```python
from build123d import *

# Parameters (mm, degrees)
F0_W     = 127
F0_H     = 190.5
F1_DEPTH = 81.28
F3_DEPTH = 91.44
F4_W     = 96.52
F4_H     = 60.96
F5_DEPTH = 60.96
F7_DEPTH = 60.96


with BuildPart() as f1:
    # F0 (on Top) → F1 (new body)
    with BuildSketch(Plane.XY):
        with Locations((-0.216242, 22.958302)):
            Rectangle(F0_W, F0_H)
    extrude(amount=F1_DEPTH)

    # F2 (on face) → F3 (cut)
    with BuildSketch(Plane.XZ.offset(72.291698)):
        Polygon((40.423758, 81.28), (-40.856242, 81.28), (-0.216242, 40.64), align=None)
    extrude(amount=-F3_DEPTH, mode=Mode.SUBTRACT)

    # F4 (on face) → F5 (join)
    with BuildSketch(Plane.XY.offset(81.28)):
        with Locations((-15.456242, 87.728302)):
            Rectangle(F4_W, F4_H)
    extrude(amount=F5_DEPTH)

    # F6 (on face) → F7 (cut)
    with BuildSketch(Plane.XZ.offset(-57.248302)):
        Polygon((-63.716242, 142.24), (-63.716242, 81.28), (-45.936242, 142.24), align=None)
        Polygon((15.023758, 142.24), (32.803758, 81.28), (32.803758, 142.24), align=None)
    extrude(amount=-F7_DEPTH, mode=Mode.SUBTRACT)


solid = f1.part
```
Can you work these out from the model? Positions are in its coordinate system, mm. A direction names the side the tool comes from. Give positions to 0.01 mm unless a question says otherwise; leave off trailing zeros. Write each loop counter-clockwise with the first axis right and the second up, starting at its lowest first coordinate (ties: lowest second). Pieces come first, ordered by that corner, then holes. Notation, with made-up numbers: (-40, 78) - (10, 78) arc R16 cw to (10, 96) - close; hole circle Ø11 at (2.25, 23). An arc over 180 degrees is marked (long way). Write item = value, one per line. Start each with the question number.
1. Imagine slicing it at B-B (z = 79). Please give me the cut outline in (x, y), and give its area (3 significant figures).
2. Imagine slicing it at A-A (y = -46.5). Please give me the cut outline in (x, z).
3. For pin 1 (5 mm diameter, centred on x = 11, y = -29, fed in from +Z), with a flat end and sliding along its axis, tell me the tip position at first contact or that it passes through.
4. On a 3-axis mill with a long thin cutter (end or side, diameter ignored), from which of +Z, -Z, +X, -X, +Y, -Y can I reach the whole of each face in a straight line? I mean faces 4 (the face through (13, 24, 81.28)), 5 (the face through (-16, 57.248, 111)), 6 (the face through (-1, 19.148, 66)). Say none if no direction works.
5. Please list where these lines run through material, in increasing order: line 1 (Y direction, x = -40, z = 135); line 2 (Z direction, x = 55.5, y = 96.5); line 3 (X direction, y = -53, z = 73).
6. Imagine slicing it at C-C (x = 44). Please give me the cut outline in (y, z), and give its area (3 significant figures).
7. Imagine slicing it at D-D (y = 68.5). Please give me the cut outline in (x, z), and give its area (3 significant figures).
8. Thinking about a two-plate mould opening in X: for faces 1 (the face through (19.819, -27.212, 60.676)), 2 (the face through (-1, 24, 0)), 3 (the face through (63.284, 22, 40)), which applies, released by +X, released by -X, zero draft, split by the parting line, or undercut?
Worked answers:
q1.outline = (-63.72, -72.29) - (-38.58, -72.29) - (-38.58, 19.15) - (38.14, 19.15) - (38.14, -72.29) - (63.28, -72.29) - (63.28, 118.21) - (-63.72, 118.21) - close
q1.area = 17,200 mm2
q2.outline = (-63.72, 0) - (63.28, 0) - (63.28, 81.28) - (40.42, 81.28) - (-0.22, 40.64) - (-40.86, 81.28) - (-63.72, 81.28) - close
q3.pin_1 = 54.36
q4.face_4 = +Z, +X, -Y
q4.face_5 = +Z, +X, -X, -Y
q4.face_6 = +Z, -Y
q5.line_1 = 57.25 to 118.21
q5.line_2 = 0 to 81.28
q5.line_3 = -63.72 to -32.58, 32.14 to 63.28
q6.outline = (-72.29, 0) - (118.21, 0) - (118.21, 81.28) - (-72.29, 81.28) - close
q6.area = 15,500 mm2
q7.outline = (-63.72, 0) - (63.28, 0) - (63.28, 81.28) - (32.8, 81.28) - (15.02, 142.24) - (-45.94, 142.24) - (-63.72, 81.28) - close
q7.area = 15,100 mm2
q8.face_1 = undercut
q8.face_2 = zero draft
q8.face_3 = released by +X
